Autodesk Inventor part; units mm, degrees
ref_plane "YZ Plane" through (0, 0, 0) normal (1, 0, 0) x (0, 1, 0)
ref_plane "XZ Plane" through (0, 0, 0) normal (0, 1, 0) x (-1, 0, 0)
ref_plane "XY Plane" through (0, 0, 0) normal (0, 0, 1) x (1, 0, 0)
sketch "Sketch1" plane through (0, 0, 0) normal (0, 0, 1) x (1, 0, 0)
  line L0 (-26.67, 0) -> (26.67, 0)
  line L1 (0, -26.67) -> (0, 26.67)
  line L2 (-19.05, 19.05) -> (-19.05, -19.05)
  line L3 (-19.05, -19.05) -> (19.05, -19.05)
  line L4 (19.05, -15.875) -> (-15.875, -15.875)
  line L5 (-15.875, -15.875) -> (-15.875, 19.05)
  line L6 (-19.05, 19.05) -> (-15.875, 19.05)
  line L7 (19.05, -19.05) -> (19.05, -15.875)
  point P0 (0, 0)
  point P1 (-19.05, 0)
  point P2 (0, -19.05)
  dimension "d0" = 38.1
  dimension "d1" = 3.175
extrude "Extrusion1" add sketch "Sketch1" along normal mid plane 482.6 contours L2 L6 L5 L0 | L0 L5 L4 L1 L3 L2 | L1 L4 L7 L3
sketch "Sketch2" plane through (-15.875, -15.875, 241.3) normal (0, 1, 0) x (1, 0, 0)
  line L0 (0, 0) -> (34.925, 0)
  line L1 (34.925, 482.6) -> (34.925, 0)
  line L2 (0, 482.6) -> (0, 0)
  line L3 (-3.175, 0) -> (-3.175, 482.6)
  line L4 (-3.175, 0) -> (34.925, 38.1)
  line L5 (34.925, 241.3) -> (0, 241.3) construction
  line L6 (-3.175, 482.6) -> (34.925, 444.5)
  line L7 (-3.175, 482.6) -> (34.925, 482.6)
  line L8 (34.925, 482.6) -> (34.925, 444.5)
  line L9 (-3.175, 0) -> (34.925, 0)
  line L10 (34.925, 0) -> (34.925, 38.1)
  point P0 (15.875, 241.3)
  dimension "d4" = 45
extrude "Extrusion2" cut sketch "Sketch2" along normal through all both and the other way through all contours L2 L4 L1 L0 | L9 L4 L2 | L6 L7 L2 | L2 L7 L1 L6
properties part number "angle template al-6061 1x1x0.125" material "Aluminum-6061"
Read the model definition and answer for the solid it produces. Units are mm, in the model's axes. A direction names the side the tool comes from. Round coordinates to 2 decimals unless told otherwise and drop trailing zeros. Write each loop counter-clockwise with the first axis right and the second up, starting at its lowest first coordinate (ties: lowest second). Pieces come first, ordered by that corner, then holes. Notation, with made-up numbers: (-26, 71.25) -> (-7, 71.25) arc R34 ccw to (-7, 104.25) -> close; hole circle Ø6 at (2.25, -1.75). An arc over 180 degrees is marked (long way). Answer in a Markdown table with one row per item. Add a question column.
1) Find section B-B, the plane x = 6. Determine the outline of the cut face in (y, z) (3 decimals), and give its area (3 significant figures).
2) Find section A-A, the plane z = 68. Determine the outline of the cut face in (x, y) (3 decimals).
3) Which of the six approach directions +Z, -Z, +X, -X, +Y, -Y give full straight-line access (tool end or side, diameter ignored) to faces 1 (the face through (-8.56, -17.02, -230.81)), 2 (the face through (-15.875, 1, -3))?
4) Given P1, Ø17.5, axis at x = -4.5, z = 0, coming from the +Y side (3 decimals); P2, Ø12, axis at x = -9.5, y = 1, coming from the +Z side; P3, Ø12, axis at x = -3, y = -12, coming from the -Z side; P4, Ø2, axis at y = -2.5, z = -111.5, coming from the +X side (3 decimals), each flat-ended and moving along its own axis, determine where each tip first touches the part or whether it passes through.
5) Find section C-C, the plane y = 0. Determine the outline of the cut face in (x, z) (3 decimals).
6) Determine the mould class of faces 3 (the face through (-8.56, -17.02, 230.81)), 4 (the face through (2, -15.875, -3)), 5 (the face through (0, -19.05, -3)) for opening direction Y: pulls with the +Y half, pulls with the -Y half, needs draft (parallel to the pull), parting line crosses it, or undercut.
7) Consider line 1 (Y direction, x = 6, z = -159.5) (3 decimals). Determine where the line is inside the solid, lowest interval first.
Findings below:
| question | item | result |
|---|---|---|
| 1 | outline | (-19.05, -216.25) -> (-15.875, -216.25) -> (-15.875, 216.25) -> (-19.05, 216.25) -> close |
| 1 | area | 1,370 mm² |
| 2 | outline | (-19.05, -19.05) -> (19.05, -19.05) -> (19.05, -15.875) -> (-15.875, -15.875) -> (-15.875, 19.05) -> (-19.05, 19.05) -> close |
| 3 | face 1 | -Z, +X, +Y, -Y |
| 3 | face 2 | +Z, -Z, +X, +Y |
| 4 | P1 | y = -15.875 |
| 4 | P2 | through |
| 4 | P3 | z = -229.83 |
| 4 | P4 | x = -15.875 |
| 5 | outline | (-19.05, -241.3) -> (-15.875, -238.125) -> (-15.875, 238.125) -> (-19.05, 241.3) -> close |
| 6 | face 3 | needs draft |
| 6 | face 4 | pulls with the +Y half |
| 6 | face 5 | pulls with the -Y half |
| 7 | line 1 | -19.05 to -15.875 |
